Verification items for the finished model (mm, model axes). Round coordinates to 2 decimals unless told otherwise and drop trailing zeros. Loops run counter-clockwise (first coordinate to the right, second up) from the corner with the lowest first, then second, coordinate; pieces in that order, holes last. Notation, with made-up numbers: (-7, 21) - (51, 21) arc R24 cw to (51, 35) - close; hole circle Ø11 at (74, 20). An arc over 180 degrees is marked (long way). Use CSV: the item, a comma, the result in double quotes.
```python
from build123d import *

# Parameters (mm, degrees)
SKETCH1_R           = 1
BOSS_EXTRUDE1_DEPTH = 27.8


with BuildPart() as part:
    # Sketch1 → Boss-Extrude1 (new body)
    with BuildSketch(Plane(origin=(0, 0, 0), x_dir=(1, 0, 0), z_dir=(0, 1, 0))):
        with Locations(Location((0, 0, 0), (0, 0, 270))):
            Circle(SKETCH1_R)
    extrude(amount=BOSS_EXTRUDE1_DEPTH)

    # Sketch4 → M1.6x0.35 Tapped Hole1 (revolve, cut)
    with BuildSketch(Plane(origin=(0, 27.8, 0), x_dir=(0, 0, 1), z_dir=(1, 0, 0))):
        Polygon((0, 0), (0, 6.375537887), (0.625, 6), (0.625, 0), align=None)
    m1_6x0_35_tapped_hole1 = revolve(axis=Axis((0, 34.15, 0), (0, -1, 0)), mode=Mode.SUBTRACT)

    # Mirror1: M1.6x0.35 Tapped Hole1 across plane
    add(m1_6x0_35_tapped_hole1.mirror(Plane(origin=(0, 13.9, 0), x_dir=(0, 0, 1), z_dir=(0, -1, 0))), mode=Mode.SUBTRACT)


solid = part.part
```
1) Mould release check, pull along X, two halves, no side actions. Record for faces 1 (the face through (0.11, 21.49, -0.02)), 2 (the face through (0.61, 24.84, -0.14)), 3 (the face through (-1, 14, 0)): +X half, -X half, draft (parallel to the pull), parting line (faces both ways), or undercut.
Returned:
face 1,"undercut"
face 2,"undercut"
face 3,"parting line"
2) Cross-section at A-A, the plane y = 25. Record the cut outline in (x, z) (3 decimals).
Returned:
outline,"circle Ø2 at (0, 0); hole circle Ø1.25 at (0, 0)"
3) Thickness scan on probe 1 along X at (y, z) = (1.4, 0) (3 decimals); probe 2 along Z at (x, y) = (0.1, 6.5); probe 3 along Z at (x, y) = (-0.2, 25.5). Record the ranges inside material, lowest first. Write a range as [from, to].
Returned:
probe 1,"x = [-1, -0.625], [0.625, 1]"
probe 2,"z = [-0.99, 0.99]"
probe 3,"z = [-0.98, -0.59], [0.59, 0.98]"
4) Cross-section at B-B, the plane y = 18.75. Record the cut outline in (x, z).
Returned:
outline,"circle Ø2 at (0, 0)"
